Geometry: final body of the model. Coordinates: model frame, mm. Face numbers are marked on the shaded views. Round coordinates to 2 decimals unless told otherwise and drop trailing zeros. Loops run counter-clockwise (first coordinate to the right, second up) from the corner with the lowest first, then second, coordinate; pieces in that order, holes last. Notation, with made-up numbers: M 12,10 L 58,10 A28 cw 58,38 Z; hole C 3.25,-14 d1. An arc over 180 degrees is marked long. Answer as a JSON object with one key per item and string values.
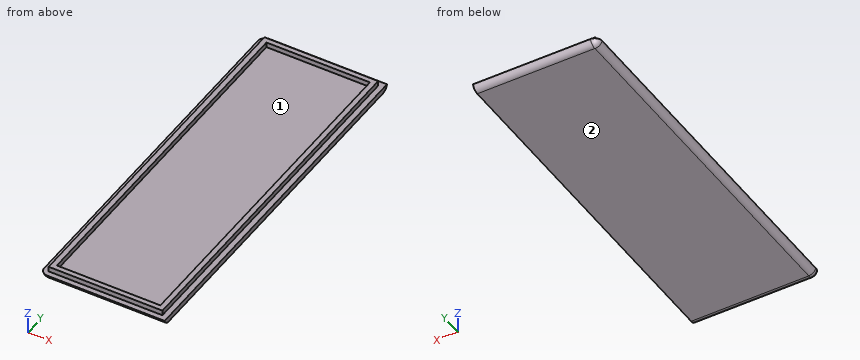
```python
from build123d import *

# Parameters (mm, degrees)
ESQUISSE1_W        = 34
ESQUISSE1_H        = 100.65
BOSS_EXTRU_1_DEPTH = 1.5
ESQUISSE2_W        = 31
ESQUISSE2_H        = 97.65
ESQUISSE2_W_2      = 28.2
ESQUISSE2_H_2      = 94.85
BOSS_EXTRU_2_DEPTH = 1.4
CONG_6_R           = 2
CONG_8_R           = 2
CONG_9_R           = 2


with BuildPart() as part:
    # Esquisse1 → Boss.-Extru.1 (new body)
    with BuildSketch(Plane.XY):
        with Locations((17, 50.325)):
            Rectangle(ESQUISSE1_W, ESQUISSE1_H)
    extrude(amount=BOSS_EXTRU_1_DEPTH)

    # Esquisse2 → Boss.-Extru.2 (add)
    with BuildSketch(Plane.XY.offset(1.5)):
        with Locations((17, 50.325)):
            Rectangle(ESQUISSE2_W, ESQUISSE2_H)
        with Locations((17, 50.325)):
            Rectangle(ESQUISSE2_W_2, ESQUISSE2_H_2, mode=Mode.SUBTRACT)
    extrude(amount=BOSS_EXTRU_2_DEPTH)

    # Congé6
    cong_6_edges = [part.edges().sort_by_distance(p)[0] for p in [
        (0, 0, 0.75),
    ]]
    fillet(cong_6_edges, radius=CONG_6_R)

    # Congé8
    cong_8_edges = [part.edges().sort_by_distance(p)[0] for p in [
        (0, 100.65, 0.75),
    ]]
    fillet(cong_8_edges, radius=CONG_8_R)

    # Congé9
    # the kernel refuses this fillet: 2 mm, written as the material it takes off along each edge
    with BuildSketch(Plane(origin=(38.841229183, 100.65, 0), x_dir=(0, -1, 0), z_dir=(-1, 0, 0)), Plane(origin=(2, 0, 0), x_dir=(0, 1, 0), z_dir=(1, 0, 0))) as cong_9_piece_1:
        with BuildLine():
            CenterArc((1.936491673, 2), CONG_9_R, 194.477512186, 75.522487814)
            Line((0, 1.5), (-0.038729833, 1.49))
            ThreePointArc((-0.038729833, 1.49), (-0.04, 0.75), (-0.04, 0))
            Line((-0.04, 0), (0, -0.04))
            Line((0, -0.04), (1.936491673, -0.04))
            Line((1.936491673, -0.04), (1.936491673, 0))
        make_face()
    extrude(amount=36.841229183, mode=Mode.SUBTRACT)
    with BuildSketch(Plane(origin=(2, 98.65, 0), x_dir=(-1, 0, 0), z_dir=(0, -1, 0))) as cong_9_piece_2:
        with BuildLine():
            CenterArc((0.063508327, -2), CONG_9_R, 14.477512186, 75.522487814)
            Line((2, -1.5), (2.038729833, -1.49))
            ThreePointArc((2.038729833, -1.49), (2.04, -0.75), (2.04, 0))
            Line((2.04, 0), (2, 0.04))
            Line((2, 0.04), (0.063508327, 0.04))
            Line((0.063508327, 0.04), (0.063508327, 0))
        make_face()
    revolve(axis=Axis((2, 98.65, 0), (0, 0, -1)), revolution_arc=90, mode=Mode.SUBTRACT)
    with BuildSketch(Plane(origin=(0, 98.65, 0), x_dir=(1, 0, 0), z_dir=(0, -1, 0))) as cong_9_piece_3:
        with BuildLine():
            CenterArc((1.936491673, 2), CONG_9_R, 194.477512186, 75.522487814)
            Line((0, 1.5), (-0.038729833, 1.49))
            ThreePointArc((-0.038729833, 1.49), (-0.04, 0.75), (-0.04, 0))
            Line((-0.04, 0), (0, -0.04))
            Line((0, -0.04), (1.936491673, -0.04))
            Line((1.936491673, -0.04), (1.936491673, 0))
        make_face()
    extrude(amount=96.65, mode=Mode.SUBTRACT)
    with BuildSketch(Plane(origin=(2, 2, 0), x_dir=(0, -1, 0), z_dir=(1, 0, 0))) as cong_9_piece_4:
        with BuildLine():
            CenterArc((0.063508327, -2), CONG_9_R, 14.477512186, 75.522487814)
            Line((2, -1.5), (2.038729833, -1.49))
            ThreePointArc((2.038729833, -1.49), (2.04, -0.75), (2.04, 0))
            Line((2.04, 0), (2, 0.04))
            Line((2, 0.04), (0.063508327, 0.04))
            Line((0.063508327, 0.04), (0.063508327, 0))
        make_face()
    revolve(axis=Axis((2, 2, 0), (0, 0, -1)), revolution_arc=90, mode=Mode.SUBTRACT)


solid = part.part
```
1) Line query: probe 1 along Y at (x, z) = (15, 1.8); probe 2 along X at (y, z) = (18.5, 2.35); probe 3 along Z at (x, y) = (23.5, 80). Output: solid intervals per line, ascending.
Geometry results:
{"probe 1": "1.5 to 2.9, 97.75 to 99.15", "probe 2": "1.5 to 2.9, 31.1 to 32.5", "probe 3": "0 to 1.5"}
2) Cut plane A-A on z = 2.35. Return the cut outline in (x, y), and give its area (3 significant figures).
Geometry results:
{"outline": "M 1.5,1.5 L 32.5,1.5 L 32.5,99.15 L 1.5,99.15 Z; hole M 2.9,2.9 L 31.1,2.9 L 31.1,97.75 L 2.9,97.75 Z", "area": "352 mm2"}
3) Cut plane B-B on x = 16. Return the cut outline in (y, z).
Geometry results:
{"outline": "M 0,1.5 A2 ccw 1.94,0 L 98.71,0 A2 ccw 100.65,1.5 L 99.15,1.5 L 99.15,2.9 L 97.75,2.9 L 97.75,1.5 L 2.9,1.5 L 2.9,2.9 L 1.5,2.9 L 1.5,1.5 Z"}
4) Pull-direction query (X, two-part tool) for the marked faces 1 and 2; classes: +X half, -X half, draft (parallel to the pull), parting line (faces both ways), or undercut.
Geometry results:
{"face 1": "undercut", "face 2": "draft"}
5) Cut plane C-C on y = 59. Return the cut outline in (x, z), and give its area (3 significant figures).
Geometry results:
{"outline": "M 0,1.5 A2 ccw 1.94,0 L 34,0 L 34,1.5 L 32.5,1.5 L 32.5,2.9 L 31.1,2.9 L 31.1,1.5 L 2.9,1.5 L 2.9,2.9 L 1.5,2.9 L 1.5,1.5 Z", "area": "54.2 mm2"}
6) First-contact query: pin 1 (1.5 mm diameter, centred on x = 24, y = 49.5, fed in from +Z); pin 2 (1.5 mm diameter, centred on x = 23.5, z = 2, fed in from -Y); pin 3 (0.7 mm diameter, centred on y = 72, z = 2, fed in from +X); pin 4 (0.7 mm diameter, centred on y = 67.5, z = 2, fed in from -X). Flat tips, straight axial feed; report the tip coordinate or a pass-through.
Geometry results:
{"pin 1": "z = 1.5", "pin 2": "y = 0", "pin 3": "x = 32.5", "pin 4": "x = 1.5"}
